Verification items for the finished model (mm, model axes). Face numbers are marked on the shaded views. A direction names the side the tool comes from. Round coordinates to 2 decimals unless told otherwise and drop trailing zeros. Write each loop counter-clockwise with the first axis right and the second up, starting at its lowest first coordinate (ties: lowest second). Pieces come first, ordered by that corner, then holes. Notation, with made-up numbers: M 64.5,34.5 L 85.5,34.5 A17 cw 85.5,64.5 Z; hole C 86.25,22.5 d1. An arc over 180 degrees is marked long. One line per item, written item: value. Start each with the question number.
Item 1: Section check C-C, the plane x = -8. Record the cut outline in (y, z).
Item 2: Tool access check on the marked faces 5, 6 and 7. Record the directions out of +Z, -Z, +X, -X, +Y, -Y that give a thin tool (end or side, any length) a straight path to the whole face; none if there is none.
Item 3: Draft check along X on the marked faces 1, 2, 3 and 4. Enter one of: +X half, -X half, draft (parallel to the pull), parting line (faces both ways), or undercut.
Item 4: Section check A-A, the plane x = -3. Record the cut outline in (y, z).
Item 5: Section check B-B, the plane z = 4.5. Record the cut outline in (x, y).
Item 6: Section check D-D, the plane z = 17.75. Record the cut outline in (x, y).
Item 7: Thickness scan on probe 1 along Y at (x, z) = (9, 2.75); probe 2 along X at (y, z) = (3.5, 12.25); probe 3 along X at (y, z) = (1, 17.75). Record the ranges inside material, lowest first. Write a range as from..to.
Item 8: Gauge pin test, flat ends, axial feed: pin 1 (3 mm diameter, centred on y = 0.5, z = 12.5, fed in from -X); pin 2 (3 mm diameter, centred on y = -2, z = 12.5, fed in from +X); pin 3 (5 mm diameter, centred on x = -15, y = -0.5, fed in from -Z); pin 4 (4.5 mm diameter, centred on x = 15.67, y = 0.1, fed in from +Z). Record the tip position at first contact, or that the pin passes through.
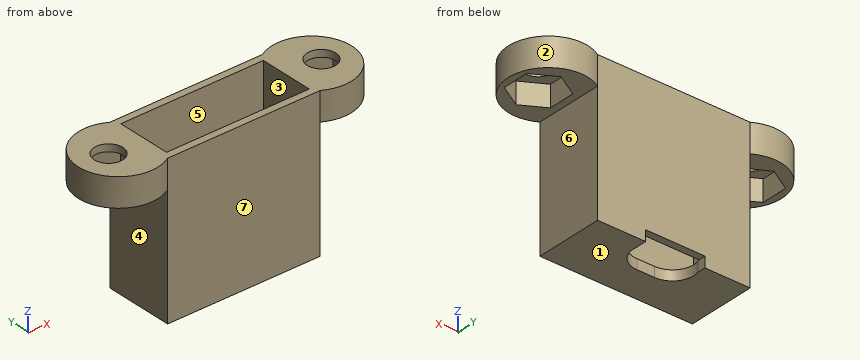
from build123d import *

# Parameters (mm, degrees)
SKETCH1_W           = 21.5
SKETCH1_H           = 9.65
BOSS_EXTRUDE1_DEPTH = 21
SKETCH3_W           = 20.1
SKETCH3_H           = 7.65
CUT_EXTRUDE1_DEPTH  = 19.6
CUT_EXTRUDE2_DEPTH  = 19.6
BOSS_EXTRUDE2_DEPTH = 4
CUT_EXTRUDE3_DEPTH  = 3
SKETCH22_R          = 2
CUT_EXTRUDE4_DEPTH  = 3
BOSS_EXTRUDE3_DEPTH = 4
CUT_EXTRUDE5_DEPTH  = 3
SKETCH25_R          = 2
CUT_EXTRUDE6_DEPTH  = 3
SKETCH26_W          = 8.360194132
SKETCH26_H          = 1.498091199
CUT_EXTRUDE7_DEPTH  = 2


with BuildPart() as part:
    # Sketch1 → Boss-Extrude1 (new body)
    with BuildSketch(Plane.XY):
        with Locations((0.67161215, 0.10146028)):
            Rectangle(SKETCH1_W, SKETCH1_H)
    extrude(amount=BOSS_EXTRUDE1_DEPTH)

    # Sketch3 → Cut-Extrude1 (cut)
    with BuildSketch(Plane.XY.offset(21)):
        with Locations((0.67161215, 0.10146028)):
            Rectangle(SKETCH3_W, SKETCH3_H)
    extrude(amount=-CUT_EXTRUDE1_DEPTH, mode=Mode.SUBTRACT)

    # Sketch5 → Cut-Extrude2 (cut)
    with BuildSketch(Plane.XY.offset(1.4)):
        with BuildLine():
            Line((-0.82838785, 5.92646028), (1.67161215, 5.92646028))
            ThreePointArc((1.67161215, 5.92646028), (4.67161215, 2.92646028), (1.67161215, -0.07353972))
            Line((1.67161215, -0.07353972), (-0.82838785, -0.07353972))
            ThreePointArc((-0.82838785, -0.07353972), (-3.82838785, 2.92646028), (-0.82838785, 5.92646028))
        make_face()
    extrude(amount=-CUT_EXTRUDE2_DEPTH, mode=Mode.SUBTRACT)

    # Sketch20 → Boss-Extrude2 (add)
    with BuildSketch(Plane.XY.offset(21)):
        with BuildLine():
            Line((-10.07838785, -4.72353972), (-10.07838785, 4.92646028))
            ThreePointArc((-10.07838785, 4.92646028), (-18.57838785, 0.10146028), (-10.07838785, -4.72353972))
        make_face()
    extrude(amount=-BOSS_EXTRUDE2_DEPTH)

    # Sketch21 → Cut-Extrude3 (cut)
    with BuildSketch(Plane(origin=(0, 0, 17), x_dir=(-1, 0, 0), z_dir=(0, 0, -1))):
        Polygon((14.32838785, 3.85146028), (11.080792586, 1.97646028), (11.080792586, -1.77353972), (14.32838785, -3.64853972), (17.575983115, -1.77353972), (17.575983115, 1.97646028), align=None)
    extrude(amount=-CUT_EXTRUDE3_DEPTH, mode=Mode.SUBTRACT)

    # Sketch22 → Cut-Extrude4 (cut)
    with BuildSketch(Plane(origin=(0, 0, 20), x_dir=(-1, 0, 0), z_dir=(0, 0, -1))):
        with Locations((14.32838785, 0.10146028)):
            Circle(SKETCH22_R)
    extrude(amount=-CUT_EXTRUDE4_DEPTH, mode=Mode.SUBTRACT)

    # Sketch23 → Boss-Extrude3 (add)
    with BuildSketch(Plane.XY.offset(21)):
        with BuildLine():
            Line((11.42161215, 4.92646028), (11.42161215, -4.72353972))
            ThreePointArc((11.42161215, -4.72353972), (19.92161215, 0.10146028), (11.42161215, 4.92646028))
        make_face()
    extrude(amount=-BOSS_EXTRUDE3_DEPTH)

    # Sketch24 → Cut-Extrude5 (cut)
    with BuildSketch(Plane(origin=(0, 0, 17), x_dir=(-1, 0, 0), z_dir=(0, 0, -1))):
        Polygon((-15.67161215, 3.85146028), (-18.919207414, 1.97646028), (-18.919207414, -1.77353972), (-15.67161215, -3.64853972), (-12.424016885, -1.77353972), (-12.424016885, 1.97646028), align=None)
    extrude(amount=-CUT_EXTRUDE5_DEPTH, mode=Mode.SUBTRACT)

    # Sketch25 → Cut-Extrude6 (cut)
    with BuildSketch(Plane(origin=(0, 0, 20), x_dir=(-1, 0, 0), z_dir=(0, 0, -1))):
        with Locations((-15.67161215, 0.10146028)):
            Circle(SKETCH25_R)
    extrude(amount=-CUT_EXTRUDE6_DEPTH, mode=Mode.SUBTRACT)

    # Sketch26 → Cut-Extrude7 (cut)
    with BuildSketch(Plane(origin=(0, 4.92646028, 0), x_dir=(1, 0, 0), z_dir=(0, 1, 0))):
        with Locations((0.472258252, -0.7490456)):
            Rectangle(SKETCH26_W, SKETCH26_H)
    extrude(amount=-CUT_EXTRUDE7_DEPTH, mode=Mode.SUBTRACT)


solid = part.part
Response values:
1. outline: M -4.72,0 L 4.93,0 L 4.93,21 L 3.93,21 L 3.93,1.4 L -3.72,1.4 L -3.72,21 L -4.72,21 Z
2. face 5: +Z
2. face 6: -Z, +X, +Y, -Y
2. face 7: +Z, -Z, -Y
3. face 1: draft
3. face 2: undercut
3. face 3: undercut
3. face 4: -X half
4. outline: M -4.72,0 L 0.86,0 L 0.86,1.4 L -3.72,1.4 L -3.72,21 L -4.72,21 Z; M 3.93,1.5 L 4.93,1.5 L 4.93,21 L 3.93,21 Z
5. outline: M -10.08,-4.72 L 11.42,-4.72 L 11.42,4.93 L -10.08,4.93 Z; hole M -9.38,-3.72 L 10.72,-3.72 L 10.72,3.93 L -9.38,3.93 Z
6. outline: M -10.08,-4.72 L 11.42,-4.72 A5.62 ccw long 11.42,4.93 L -10.08,4.93 A5.62 ccw long Z; hole M -17.58,-1.77 L -14.33,-3.65 L -11.08,-1.77 L -11.08,1.98 L -14.33,3.85 L -17.58,1.98 Z; hole M -9.38,-3.72 L 10.72,-3.72 L 10.72,3.93 L -9.38,3.93 Z; hole M 12.42,-1.77 L 15.67,-3.65 L 18.92,-1.77 L 18.92,1.98 L 15.67,3.85 L 12.42,1.98 Z
7. probe 1: y = -4.72..-3.72, 3.93..4.93
7. probe 2: x = -10.08..-9.38, 10.72..11.42
7. probe 3: x = -18.51..-17.58, -11.08..-9.38, 10.72..12.42, 18.92..19.85
8. pin 1: stops at x = -10.08
8. pin 2: stops at x = 11.42
8. pin 3: stops at z = 17
8. pin 4: stops at z = 21
